from build123d import *

# Parameters (mm, degrees)
F0_R     = 57.15
F1_DEPTH = 6.35
F2_R     = 42.926
F3_DEPTH = 4.7752
F4_SIZE  = 0.762
F6_D     = 7.112
F8_D     = 9.525


with BuildPart() as f1:
    # F0 (on Right) → F1 (new body)
    with BuildSketch(Plane.YZ):
        Circle(F0_R)
    extrude(amount=F1_DEPTH)

    # F2 (on face) → F3 (join)
    with BuildSketch(Plane(origin=(0, 0, 0), x_dir=(0, -1, 0), z_dir=(-1, 0, 0))):
        Circle(F2_R)
    extrude(amount=F3_DEPTH)

    # F4
    f4_edges = [f1.edges().sort_by_distance(p)[0] for p in [
        (6.35, -57.15, 0),
        (0, -57.15, 0),
        (-4.7752, 42.926, 0),
    ]]
    chamfer(f4_edges, length=F4_SIZE)

    # F6 (through all)
    with Locations(Plane.YZ.offset(6.35)):
        with Locations((0, 49.276), (49.276, 0), (0, -49.276), (-49.276, 0)):
            Hole(F6_D / 2)

    # F8 (through all)
    with Locations(Plane.YZ.offset(6.35)):
        with Locations((0, 22.225), (0, -22.225)):
            Hole(F8_D / 2)


solid = f1.part
Geometry check sheet. Reference: the model listing, model coordinates, mm. A direction names the side the tool comes from. Give positions to 0.01 mm unless a question says otherwise; leave off trailing zeros. Order: outer loops, then holes, each group sorted by start corner. A loop starts at its lowest first (then second) coordinate and runs counter-clockwise, first axis right, second up. Notation, with made-up numbers: (28.5, 89) - (36.5, 89) arc R12 cw to (36.5, 108) - close; hole circle Ø5 at (54.5, -19). An arc over 180 degrees is marked (long way). Use one line per item in the form item = value.
1) Draft check along Z on faces 1 (the face through (-4.775, 1, 1)), 2 (the face through (-1.979, -40.944, 12.894)), 3 (the face through (3.131, -52.668, 1.068)). Enter one of: released by +Z, released by -Z, zero draft, split by the parting line, or undercut.
Working result:
face_1 = zero draft
face_2 = split by the parting line
face_3 = undercut
2) Depth check by flat-ended pin: pin 1 Ø5 at (x, z) = (0.5, 42) entering from -Y; pin 2 Ø4 at (x, z) = (3, 17) entering from +Y; pin 3 Ø1.5 at (x, y) = (0.5, 11.5) entering from +Z; pin 4 Ø4.5 at (y, z) = (0, 49.276) entering from +X. Enter the tip coordinate at first touch or a pass-through.
Working result:
pin_1 = -41.29
pin_2 = 55.15
pin_3 = 56.12
pin_4 = through
3) Sectioned sample at B-B (z = 0). Record the boundary of the cut face in (x, y).
Working result:
outline = (-4.78, -42.16) - (-4.01, -42.93) - (0, -42.93) - (0, -45.72) - (6.35, -45.72) - (6.35, 45.72) - (0, 45.72) - (0, 42.93) - (-4.01, 42.93) - (-4.78, 42.16) - close; (0, -56.39) - (0.76, -57.15) - (5.59, -57.15) - (6.35, -56.39) - (6.35, -52.83) - (0, -52.83) - close; (0, 52.83) - (6.35, 52.83) - (6.35, 56.39) - (5.59, 57.15) - (0.76, 57.15) - (0, 56.39) - close
4) Access from +Z, -Z, +X, -X, +Y, -Y to the whole of each face (thin tool, end or side, straight path). Record for faces 4 (the face through (6.35, -1, 1)), 5 (the face through (0, -13, -42)).
Working result:
face_4 = +Z, -Z, +X, +Y, -Y
face_5 = -X
5) Material ranges on probe 1 along Z at (x, y) = (3.75, 0); probe 2 along Y at (x, z) = (5, 3); probe 3 along Y at (x, z) = (2, -2.5), recorded low to high. Write a range as from..to.
Working result:
probe_1 = -57.15..-52.83, -45.72..-26.99, -17.46..17.46, 26.99..45.72, 52.83..57.15
probe_2 = -57.07..-51.19, -47.37..47.37, 51.19..57.07
probe_3 = -57.1..-51.8, -46.75..46.75, 51.8..57.1
6) Sectioned sample at A-A (y = 0). Count the separate pieces of the cut face and the enclosed holes in it, and give its area (3 significant figures).
Working result:
separate_pieces = 5
enclosed_holes = 0
area = 832 mm^2
